Check sheet for the drawn part. Datum: minimum x, y, z corner. Units: mm. A direction names the side the tool comes from. Coordinates: 2 decimals unless noted, no trailing zeros. Order: outer loops, then holes, each group sorted by start corner. A loop starts at its lowest first (then second) coordinate and runs counter-clockwise, first axis right, second up.
1. Thickness scan on line 1 (X direction, y = 19.75, z = 39); line 2 (Y direction, x = 32, z = 29); line 3 (X direction, y = 13.5, z = 37.5). Record the ranges inside material, lowest first.
2. Cross-section at D-D (z = 8). Enter the section's corners in (x, y).
3. Cross-section at B-B (y = 22.25). Enter the section's corners in (x, z), then the cut area to 3 significant figures.
4. Set-up check for the marked faces 5, 6, 7, 8 and 9: record each of +Z, -Z, +X, -X, +Y, -Y from which the full face is reachable in a straight line by a thin tool's end or side.
5. Draft check along Y on the marked faces 1, 2, 3 and 4. Enter one of: released by +Y, released by -Y, zero draft, split by the parting line, or undercut.
6. Cross-section at A-A (x = 31). Enter the section's corners in (y, z).
7. Gauge pin test, flat ends, axial feed: pin 1 Ø3.5 at (x, z) = (22, 28.5) entering from -Y; pin 2 Ø1.5 at (x, z) = (6, 22.5) entering from -Y. Record the tip position at first contact, or that the pin passes through.
8. Cross-section at C-C (z = 25). Enter the section's corners in (x, y), then the cut area to 3 significant figures.
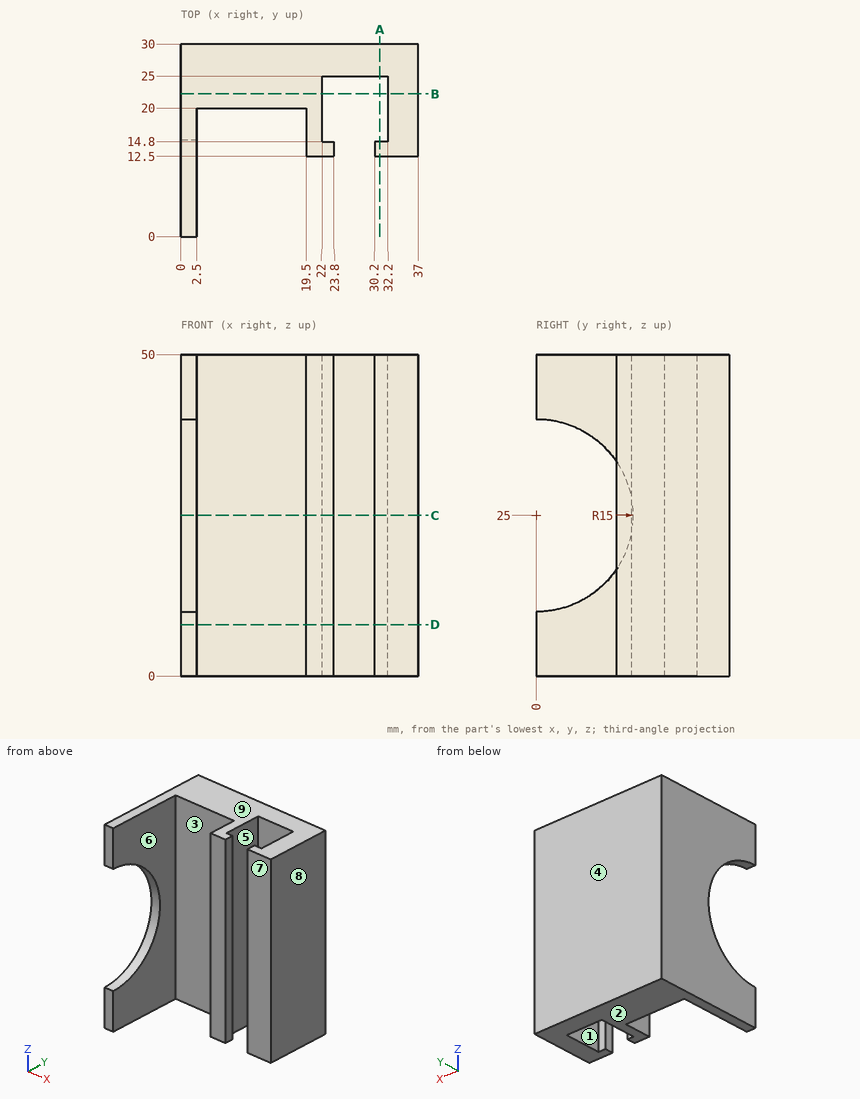
Data:
1. line 1: x = 0 to 2.5, 19.5 to 22, 32.2 to 37
1. line 2: y = 12.5 to 14.8, 25 to 30
1. line 3: x = 0 to 2.5, 19.5 to 23.8, 30.2 to 37
2. outline: (0, 0) - (2.5, 0) - (2.5, 20) - (19.5, 20) - (19.5, 12.5) - (23.8, 12.5) - (23.8, 14.8) - (22, 14.8) - (22, 25) - (32.2, 25) - (32.2, 14.8) - (30.2, 14.8) - (30.2, 12.5) - (37, 12.5) - (37, 30) - (0, 30) - close
3. outline: (0, 0) - (22, 0) - (22, 50) - (0, 50) - close; (32.2, 0) - (37, 0) - (37, 50) - (32.2, 50) - close
3. area: 1,340 mm2
4. face 5: +Z, -Z
4. face 6: +Z, -Z, -Y
4. face 7: +Z, -Z, +X, -Y
4. face 8: +Z, -Z, +X, +Y, -Y
4. face 9: +Z, +X, -X, +Y, -Y
5. face 1: undercut
5. face 2: zero draft
5. face 3: released by -Y
5. face 4: released by +Y
6. outline: (12.5, 0) - (14.8, 0) - (14.8, 50) - (12.5, 50) - close; (25, 0) - (30, 0) - (30, 50) - (25, 50) - close
7. pin 1: stops at y = 12.5
7. pin 2: stops at y = 20
8. outline: (0, 15) - (2.5, 15) - (2.5, 20) - (19.5, 20) - (19.5, 12.5) - (23.8, 12.5) - (23.8, 14.8) - (22, 14.8) - (22, 25) - (32.2, 25) - (32.2, 14.8) - (30.2, 14.8) - (30.2, 12.5) - (37, 12.5) - (37, 30) - (0, 30) - close
8. area: 395 mm2
